Work out the finished part from the listing and answer in its coordinate system (mm). A direction names the side the tool comes from. Coordinates: 2 decimals unless noted, no trailing zeros. Loops run counter-clockwise (first coordinate to the right, second up) from the corner with the lowest first, then second, coordinate; pieces in that order, holes last. Notation, with made-up numbers: (18, 80) -> (37, 80) arc R20 ccw to (37, 119) -> close; hole circle Ø3 at (-7, -13). An arc over 180 degrees is marked (long way). Use a Markdown table: item, result.
from build123d import *

# Parameters (mm, degrees)
F0_W      = 112.4612912536
F0_H      = 62.7993419766
F1_DEPTH  = 25.4
F2_R      = 5.08
F3_W      = 78.4117951989
F3_H      = 62.7993419766
F4_DEPTH  = 25.4
F5_W      = 12.7
F5_H      = 50.8
F7_W      = 56.2817417085
F7_H      = 15.2776930481
F8_DEPTH  = 25.4
F9_W      = 12.7
F9_H      = 24.5103910565
F10_DEPTH = 25.4
F11_R     = 5.08
F12_R     = 5.08


with BuildPart() as f1:
    # F0 (on Front) → F1 (new body)
    with BuildSketch(Plane.XZ):
        Rectangle(F0_W, F0_H)
    extrude(amount=F1_DEPTH)

    # F2
    f2_edges = [f1.edges().sort_by_distance(p)[0] for p in [
        (-56.230646, -12.7, 31.399671),
        (56.230646, -12.7, 31.399671),
    ]]
    fillet(f2_edges, radius=F2_R)

    # F3 (on face) → F4 (join)
    with BuildSketch(Plane.XZ.offset(25.4)):
        with Locations((3.4460537136, 0)):
            Rectangle(F3_W, F3_H)
    extrude(amount=F4_DEPTH)

    # F5 (on face) → F6 (revolve, cut)
    with BuildSketch(Plane.XY.offset(31.3996709883)):
        with Locations((-6.35, -25.4)):
            Rectangle(F5_W, F5_H)
    revolve(axis=Axis((0, -25.4, 31.3996709883), (0, 1, 0)), mode=Mode.SUBTRACT)

    # F7 (on face) → F8 (cut)
    with BuildSketch(Plane.XZ.offset(50.8)):
        with Locations((0, -23.7608244643)):
            Rectangle(F7_W, F7_H)
    extrude(amount=-F8_DEPTH, mode=Mode.SUBTRACT)

    # F9 (on face) → F10 (cut)
    with BuildSketch(Plane.XZ.offset(50.8)):
        with Locations((-29.4098438859, 19.1444754601)):
            Rectangle(F9_W, F9_H)
        with Locations((36.301951313, 19.1444754601)):
            Rectangle(F9_W, F9_H)
    extrude(amount=-F10_DEPTH, mode=Mode.SUBTRACT)

    # F11
    f11_edges = [f1.edges().sort_by_distance(p)[0] for p in [
        (-23.059844, -38.1, 6.88928),
    ]]
    fillet(f11_edges, radius=F11_R)

    # F12
    f12_edges = [f1.edges().sort_by_distance(p)[0] for p in [
        (29.951951, -38.1, 6.88928),
    ]]
    fillet(f12_edges, radius=F12_R)


solid = f1.part
Q1. Consider line 1 (X direction, y = -44.5, z = -25); line 2 (X direction, y = -47.5, z = -14); line 3 (Y direction, x = -40, z = -28). Determine where each line is inside the solid, lowest interval first. Write a range as [from, to].
Solved:
| item | result |
|---|---|
| line 1 | [-35.76, -28.14], [28.14, 42.65] |
| line 2 | [-35.76, 42.65] |
| line 3 | [-25.4, 0] |
Q2. Section D-D on z = -2 is taken. Determine the outline of the cut face in (x, y), and give its area (3 significant figures).
Solved:
| item | result |
|---|---|
| outline | (-56.23, -25.4) -> (-35.76, -25.4) -> (-35.76, -50.8) -> (42.65, -50.8) -> (42.65, -25.4) -> (56.23, -25.4) -> (56.23, 0) -> (-56.23, 0) -> close |
| area | 4,850 mm² |
Q3. Determine the mould class of faces 1 (the flat face through (42.652, -38, -13)), 2 (the flat face through (0, -38, -16.122)), 3 (the cylindrical face through (-54.782, -12.878, 29.872)) for opening direction X: pulls with the +X half, pulls with the -X half, needs draft (parallel to the pull), parting line crosses it, or undercut.
Solved:
| item | result |
|---|---|
| face 1 | pulls with the +X half |
| face 2 | undercut |
| face 3 | pulls with the -X half |
Q4. Section A-A on y = -32.5 is taken. Determine the outline of the cut face in (x, z).
Solved:
| item | result |
|---|---|
| outline | (-35.76, -31.4) -> (-28.14, -31.4) -> (-28.14, -16.12) -> (28.14, -16.12) -> (28.14, -31.4) -> (42.65, -31.4) -> (42.65, 6.89) -> (35.03, 6.89) arc R5.08 cw to (29.95, 11.97) -> (29.95, 31.4) -> (12.7, 31.4) arc R12.7 cw to (-12.7, 31.4) -> (-23.06, 31.4) -> (-23.06, 11.97) arc R5.08 cw to (-28.14, 6.89) -> (-35.76, 6.89) -> close |
Q5. Given pin 1 Ø8 at (x, z) = (43.5, 11.5) entering from -Y; pin 2 Ø7.5 at (y, z) = (-39.5, -20) entering from -X; pin 3 Ø5 at (x, y) = (-6.5, -44.5) entering from +Z, each flat-ended and moving along its own axis, determine where each tip first touches the part or whether it passes through.
Solved:
| item | result |
|---|---|
| pin 1 | y = -25.4 |
| pin 2 | x = -35.76 |
| pin 3 | z = 22.44 |
Q6. Section B-B on z = 22.5 is taken. Determine the outline of the cut face in (x, y), and give its area (3 significant figures).
Solved:
| item | result |
|---|---|
| outline | (-56.23, -25.4) -> (-23.06, -25.4) -> (-23.06, -50.8) -> (-9.06, -50.8) -> (-9.06, 0) -> (-56.23, 0) -> close; (9.06, -50.8) -> (29.95, -50.8) -> (29.95, -25.4) -> (56.23, -25.4) -> (56.23, 0) -> (9.06, 0) -> close |
| area | 3,280 mm² |
Q7. Section C-C on x = 0 is taken. Determine the outline of the cut face in (y, z).
Solved:
| item | result |
|---|---|
| outline | (-50.8, -16.12) -> (-25.4, -16.12) -> (-25.4, -31.4) -> (0, -31.4) -> (0, 18.7) -> (-50.8, 18.7) -> close |
Q8. For faces 4 (the flat face through (-56.231, -13, -3)), 5 (the flat face through (-28.141, -38, -24)), 6 (the flat face through (-35.76, -38, -13)), 7 (the cylindrical face through (-24.508, -37.922, 8.417)), 8 (the cylindrical face through (31.4, -37.92, 8.42)), determine the directions among +Z, -Z, +X, -X, +Y, -Y from which every point of the face is accessible in a straight line to the end or side of a thin tool.
Solved:
| item | result |
|---|---|
| face 4 | +Z, -Z, -X, +Y, -Y |
| face 5 | -Z, -Y |
| face 6 | +Z, -Z, -X, -Y |
| face 7 | +Z, -X, -Y |
| face 8 | +Z, +X, -Y |
